from build123d import *

# Parameters (mm, degrees)
SKETCH1_W           = 130
SKETCH1_H           = 130
SKETCH1_W_2         = 30
SKETCH1_H_2         = 30
BOSS_EXTRUDE1_DEPTH = 3
CUT_EXTRUDE1_DEPTH  = 3
CUT_EXTRUDE2_DEPTH  = 3
SKETCH4_W           = 20
SKETCH4_H           = 3
SKETCH4_W_2         = 10
CUT_EXTRUDE3_DEPTH  = 10


with BuildPart() as part:
    # Sketch1 → Boss-Extrude1 (new body)
    with BuildSketch(Plane(origin=(0, 0, 0), x_dir=(1, 0, 0), z_dir=(0, 1, 0))):
        Rectangle(SKETCH1_W, SKETCH1_H)
        Polygon((-55, 40.857864376), (-25, 10.857864376), (-25, -10.857864376), (-55, -40.857864376), align=None, mode=Mode.SUBTRACT)
        Polygon((-40.857864376, -55), (-10.857864376, -25), (10.857864376, -25), (40.857864376, -55), align=None, mode=Mode.SUBTRACT)
        Polygon((55, -40.857864376), (25, -10.857864376), (25, 10.857864376), (55, 40.857864376), align=None, mode=Mode.SUBTRACT)
        Polygon((40.857864376, 55), (10.857864376, 25), (-10.857864376, 25), (-40.857864376, 55), align=None, mode=Mode.SUBTRACT)
        Rectangle(SKETCH1_W_2, SKETCH1_H_2, mode=Mode.SUBTRACT)
    extrude(amount=BOSS_EXTRUDE1_DEPTH)

    # Sketch2 → Cut-Extrude1 (cut)
    with BuildSketch(Plane(origin=(0, 3, 0), x_dir=(1, 0, 0), z_dir=(0, 1, 0))):
        with BuildLine():
            ThreePointArc((-55.8, 57.5), (-58.702081528, 58.702081528), (-57.5, 55.8))
            Line((-57.5, 55.8), (-57.5, 57.5))
            Line((-57.5, 57.5), (-55.8, 57.5))
        make_face()
        with BuildLine():
            Line((-57.5, 57.5), (-57.5, 55.8))
            ThreePointArc((-57.5, 55.8), (-56.297918472, 56.297918472), (-55.8, 57.5))
            Line((-55.8, 57.5), (-57.5, 57.5))
        make_face()
        with BuildLine():
            Line((-57.5, -55.8), (-57.5, -57.5))
            Line((-57.5, -57.5), (-55.8, -57.5))
            ThreePointArc((-55.8, -57.5), (-56.297918472, -56.297918472), (-57.5, -55.8))
        make_face()
        with BuildLine():
            Line((-55.8, -57.5), (-57.5, -57.5))
            Line((-57.5, -57.5), (-57.5, -55.8))
            ThreePointArc((-57.5, -55.8), (-58.702081528, -58.702081528), (-55.8, -57.5))
        make_face()
        with BuildLine():
            ThreePointArc((57.5, -55.8), (56.297918472, -56.297918472), (55.8, -57.5))
            Line((55.8, -57.5), (57.5, -57.5))
            Line((57.5, -57.5), (57.5, -55.8))
        make_face()
        with BuildLine():
            Line((57.5, -57.5), (55.8, -57.5))
            ThreePointArc((55.8, -57.5), (57.5, -59.2), (59.2, -57.5))
            ThreePointArc((59.2, -57.5), (58.702081528, -56.297918472), (57.5, -55.8))
            Line((57.5, -55.8), (57.5, -57.5))
        make_face()
        with BuildLine():
            ThreePointArc((55.8, 57.5), (56.297918472, 56.297918472), (57.5, 55.8))
            Line((57.5, 55.8), (57.5, 57.5))
            Line((57.5, 57.5), (55.8, 57.5))
        make_face()
        with BuildLine():
            Line((57.5, 57.5), (57.5, 55.8))
            ThreePointArc((57.5, 55.8), (58.702081528, 56.297918472), (59.2, 57.5))
            ThreePointArc((59.2, 57.5), (57.5, 59.2), (55.8, 57.5))
            Line((55.8, 57.5), (57.5, 57.5))
        make_face()
    extrude(amount=-CUT_EXTRUDE1_DEPTH, mode=Mode.SUBTRACT)

    # Sketch3 → Cut-Extrude2 (cut)
    with BuildSketch(Plane(origin=(0, 3, 0), x_dir=(1, 0, 0), z_dir=(0, 1, 0))):
        with BuildLine():
            Line((-22.5, -20.8), (-22.5, -22.5))
            Line((-22.5, -22.5), (-20.8, -22.5))
            ThreePointArc((-20.8, -22.5), (-21.297918472, -21.297918472), (-22.5, -20.8))
        make_face()
        with BuildLine():
            Line((-20.8, -22.5), (-22.5, -22.5))
            Line((-22.5, -22.5), (-22.5, -20.8))
            ThreePointArc((-22.5, -20.8), (-23.702081528, -23.702081528), (-20.8, -22.5))
        make_face()
        with BuildLine():
            ThreePointArc((-20.8, 22.5), (-23.702081528, 23.702081528), (-22.5, 20.8))
            Line((-22.5, 20.8), (-22.5, 22.5))
            Line((-22.5, 22.5), (-20.8, 22.5))
        make_face()
        with BuildLine():
            Line((-22.5, 22.5), (-22.5, 20.8))
            ThreePointArc((-22.5, 20.8), (-21.297918472, 21.297918472), (-20.8, 22.5))
            Line((-20.8, 22.5), (-22.5, 22.5))
        make_face()
        with BuildLine():
            ThreePointArc((22.5, -20.8), (21.297918472, -21.297918472), (20.8, -22.5))
            Line((20.8, -22.5), (22.5, -22.5))
            Line((22.5, -22.5), (22.5, -20.8))
        make_face()
        with BuildLine():
            Line((22.5, -22.5), (20.8, -22.5))
            ThreePointArc((20.8, -22.5), (22.5, -24.2), (24.2, -22.5))
            ThreePointArc((24.2, -22.5), (23.702081528, -21.297918472), (22.5, -20.8))
            Line((22.5, -20.8), (22.5, -22.5))
        make_face()
        with BuildLine():
            ThreePointArc((20.8, 22.5), (21.297918472, 21.297918472), (22.5, 20.8))
            Line((22.5, 20.8), (22.5, 22.5))
            Line((22.5, 22.5), (20.8, 22.5))
        make_face()
        with BuildLine():
            Line((22.5, 22.5), (22.5, 20.8))
            ThreePointArc((22.5, 20.8), (23.702081528, 21.297918472), (24.2, 22.5))
            ThreePointArc((24.2, 22.5), (22.5, 24.2), (20.8, 22.5))
            Line((20.8, 22.5), (22.5, 22.5))
        make_face()
    extrude(amount=-CUT_EXTRUDE2_DEPTH, mode=Mode.SUBTRACT)

    # Sketch4 → Cut-Extrude3 (cut)
    with BuildSketch(Plane.XZ):
        with Locations((40, 63.5)):
            Rectangle(SKETCH4_W, SKETCH4_H)
        with Locations((5, 63.5)):
            Rectangle(SKETCH4_W_2, SKETCH4_H)
        with Locations((-5, 63.5)):
            Rectangle(SKETCH4_W_2, SKETCH4_H)
        with Locations((-40, 63.5)):
            Rectangle(SKETCH4_W, SKETCH4_H)
    extrude(amount=-CUT_EXTRUDE3_DEPTH, mode=Mode.SUBTRACT)


solid = part.part
Verification items for the finished model (mm, model axes). A direction names the side the tool comes from. Round coordinates to 2 decimals unless told otherwise and drop trailing zeros. Loops run counter-clockwise (first coordinate to the right, second up) from the corner with the lowest first, then second, coordinate; pieces in that order, holes last. Notation, with made-up numbers: (-37, 31.25) - (-3, 31.25) arc R19 cw to (-3, 55.25) - close; hole circle Ø3 at (77, -25.75). An arc over 180 degrees is marked (long way). Use a Markdown table: item, result. Add a question column.
1. Section check D-D, the plane y = 2.5. Give the number of separate pieces and of enclosed holes in the cut face, plus the area to 3 significant figures.
2. Access from +Z, -Z, +X, -X, +Y, -Y to the whole of each face (thin tool, end or side, straight path). Record for faces 4 (the face through (40.21, 1.48, 26.07)), 5 (the face through (10, 1, 63)).
3. Section check B-B, the plane x = -34. Record the boundary of the cut face in (y, z).
4. Thickness scan on probe 1 along X at (y, z) = (0.85, 57.5); probe 2 along X at (y, z) = (2.9, 4.5). Record the ranges inside material, lowest first. Write a range as [from, to].
5. Release check for a two-part mould opening along X. For faces 1 (the face through (-50, 1, 63)), 2 (the face through (-0.9, 0, -15.4)), 3 (the face through (-65, 1, 1)) record: released by +X, released by -X, zero draft, split by the parting line, or undercut.
6. Gauge pin test, flat end, axial feed: pin 1 (1 mm diameter, centred on x = -3.5, y = 2.5, fed in from +Z). Record the tip position at first contact, or that the pin passes through.
7. Section check A-A, the plane z = 31. Record the boundary of the cut face in (x, y), plus the area to 3 significant figures.
8. Section check C-C, the plane z = -45. Record the boundary of the cut face in (x, y).
Checks:
| question | item | result |
|---|---|---|
| 1 | separate pieces | 1 |
| 1 | enclosed holes | 13 |
| 1 | area | 9,540 mm^2 |
| 2 | face 4 | +Y, -Y |
| 2 | face 5 | +Z, +Y, -Y |
| 3 | outline | (0, -65) - (3, -65) - (3, -55) - (0, -55) - close; (0, -48.14) - (3, -48.14) - (3, -19.86) - (0, -19.86) - close; (0, 19.86) - (3, 19.86) - (3, 48.14) - (0, 48.14) - close; (0, 55) - (3, 55) - (3, 62) - (0, 62) - close |
| 4 | probe 1 | x = [-65, -59.2], [-55.8, 55.8], [59.2, 65] |
| 4 | probe 2 | x = [-65, -55], [-25, -15], [15, 25], [55, 65] |
| 5 | face 1 | undercut |
| 5 | face 2 | zero draft |
| 5 | face 3 | released by -X |
| 6 | pin 1 | stops at z = 62 |
| 7 | outline | (-65, 0) - (-55, 0) - (-55, 3) - (-65, 3) - close; (-45.14, 0) - (-16.86, 0) - (-16.86, 3) - (-45.14, 3) - close; (16.86, 0) - (45.14, 0) - (45.14, 3) - (16.86, 3) - close; (55, 0) - (65, 0) - (65, 3) - (55, 3) - close |
| 7 | area | 230 mm^2 |
| 8 | outline | (-65, 0) - (-30.86, 0) - (-30.86, 3) - (-65, 3) - close; (30.86, 0) - (65, 0) - (65, 3) - (30.86, 3) - close |
